Build history of the part. All positions in model axes, mm. A direction names the side the tool comes from. Round coordinates to 2 decimals unless told otherwise and drop trailing zeros. Loops run counter-clockwise (first coordinate to the right, second up) from the corner with the lowest first, then second, coordinate; pieces in that order, holes last. Notation, with made-up numbers: (-22.75, 58) - (30.25, 58) arc R14 ccw to (30.25, 64) - close; hole circle Ø4 at (77.25, 86). An arc over 180 degrees is marked (long way). Answer as CSV lines item,"result". Start each with the question number.
Autodesk Inventor part; units mm, degrees
ref_plane "YZ Plane" through (0, 0, 0) normal (1, 0, 0) x (0, 1, 0)
ref_plane "XZ Plane" through (0, 0, 0) normal (0, 1, 0) x (-1, 0, 0)
ref_plane "XY Plane" through (0, 0, 0) normal (0, 0, 1) x (1, 0, 0)
sketch "Sketch1" plane through (0, 0, 0) normal (0, 1, 0) x (-1, 0, 0)
  line L0 (56, 0) -> (-56, 0)
  line L1 (0, -49) -> (0, 49)
  line L2 (40, -20) -> (-40, -20)
  line L3 (-40, -20) -> (-40, 20)
  line L4 (-40, 20) -> (40, 20)
  line L5 (40, 20) -> (40, -20)
  line L6 (27.5, -35) -> (-27.5, -35) construction
  line L7 (-27.5, -35) -> (-27.5, 35) construction
  line L8 (-27.5, 35) -> (27.5, 35) construction
  line L9 (27.5, 35) -> (27.5, -35) construction
  point P0 (0, 0)
  dimension "d0" = 80
  dimension "d1" = 40
  dimension "d2" = 70
  dimension "d3" = 55
extrude "Extrusion1" add sketch "Sketch1" along normal blind 4
sketch "Sketch18" plane through (0, 4, 0) normal (0, 1, 0) x (1, 0, 0)
  line L0 (40, 20) -> (-40, 20)
  line L1 (-40, 20) -> (-40, -20)
  line L2 (-40, -20) -> (40, -20)
  line L3 (40, -20) -> (40, 20)
  line L4 (-40, -20) -> (40, -20)
  line L5 (40, -20) -> (40, -17)
  line L6 (40, -17) -> (-40, -17)
  line L7 (-40, -17) -> (-40, -20)
  line L8 (-40, 20) -> (-40, -20)
  line L9 (40, -20) -> (40, 20)
  line L10 (-40, -20) -> (40, -20)
  point P0 (0, 0)
  dimension "d207" = 3
extrude "Extrusion13" add sketch "Sketch18" along normal blind 10 contours L3 L2 L1 L6
sketch "Sketch19" plane through (0, 4, 0) normal (0, 1, 0) x (1, 0, 0)
  line L0 (-40, -17) -> (40, -17)
  line L1 (40, -17) -> (40, 20)
  line L2 (40, 20) -> (-40, 20)
  line L3 (-40, 20) -> (-40, -17)
  line L4 (0, 28) -> (0, -28)
  point P0 (0, 0)
  point P1 (-30, 10)
  point P2 (30, 10)
  dimension "d210" = 10
  dimension "d211" = 10
hole "Hole9" at (-30, 4, -10) at (30, 4, -10) direction (0, -1, 0) diameter 6 end through all
sketch "Sketch20" plane through (0, 4, 0) normal (0, 1, 0) x (1, 0, 0)
  circle A0 centre (-30, 10) radius 3
  line L0 (-40, -17) -> (40, -17)
  line L1 (40, -17) -> (40, 20)
  line L2 (40, 20) -> (-40, 20)
  line L3 (-40, 20) -> (-40, -17)
  line L4 (-30, -17) -> (-30, 20) construction
  line L5 (-40, 20) -> (-40, -17)
  line L6 (40, 20) -> (-40, 20)
  line L7 (40, -17) -> (-40, -17)
  line L8 (-39.3154, 10) -> (-16.7888, 10) construction
  line L9 (0, 28) -> (0, -28)
  point P0 (0, 0)
  point P1 (-37, 10)
  point P2 (-23, 10)
  point P3 (-30, 3)
  point P4 (-30, 17)
  point P5 (37, 10)
  point P6 (23, 10)
  point P7 (30, 3)
  point P8 (30, 17)
  dimension "d219" = 7
  dimension "d220" = 7
  dimension "d221" = 7
  dimension "d222" = 7
hole "Hole10" at (-37, 4, -10) at (-23, 4, -10) at (-30, 4, -3) at (-30, 4, -17) at (30, 4, -3) at (37, 4, -10) at (30, 4, -17) at (23, 4, -10) direction (0, -1, 0) diameter 2 end through all
fillet "Fillet11" radius 10 2 edges at (40, 2, -20) (-40, 2, -20)
sketch "Sketch21" plane through (40, 4, 17) normal (0, 0, -1) x (-1, 0, 0)
  line L0 (80, 0) -> (0, 0)
  line L1 (80, 0) -> (80, 10)
  line L2 (0, 10) -> (80, 10)
  line L3 (0, 0) -> (0, 10)
  point P0 (40, -4)
  point P1 (5, 5)
  point P2 (75, 5)
  dimension "d232" = 5
  dimension "d233" = 5
  dimension "d234" = 5
  dimension "d235" = 5
hole "Hole11" at (35, 9, 17) at (-35, 9, 17) direction (0, 0, 1) diameter 3 end through all
chamfer "Chamfer5" distance 4 angle 45 2 edges at (-40, 14, 18.5) (40, 14, 18.5)
fillet "Fillet12" radius 3 4 edges at (-36, 14, 18.5) (-40, 10, 18.5) (36, 14, 18.5) (40, 10, 18.5)
sketch "Sketch22" plane through (40, 4, 17) normal (0, 0, -1) x (-1, 0, 0)
  circle A0 centre (5, 5) radius 1.5
  circle A1 centre (75, 5) radius 1.5
  arc A2 (0.8787, 6.8787) -> (0, 4.7574) centre (3, 4.7574) ccw
  line L0 (0, 0) -> (0, 4.7574)
  line L1 (80, 0) -> (0, 0)
  line L2 (80, 0) -> (80, 4.7574)
  arc A3 (80, 4.7574) -> (79.1213, 6.8787) centre (77, 4.7574) ccw
  line L3 (76.8787, 9.1213) -> (79.1213, 6.8787)
  arc A4 (76.8787, 9.1213) -> (74.7574, 10) centre (74.7574, 7) ccw
  line L4 (5.2426, 10) -> (74.7574, 10)
  arc A5 (5.2426, 10) -> (3.1213, 9.1213) centre (5.2426, 7) ccw
  line L5 (0.8787, 6.8787) -> (3.1213, 9.1213)
  line L6 (10, 0) -> (70, 0)
  line L7 (20, 10) -> (60, 10)
  line L8 (60, 10) -> (60, 0)
  line L9 (60, 0) -> (20, 0)
  line L10 (20, 0) -> (20, 10)
  point P0 (40, -4)
  point P1 (40, 5)
  dimension "d247" = 5
  dimension "d248" = 40
  dimension "d256" = 40
  dimension "d257" = 10
  dimension "d258" = 20
extrude "Extrusion14" cut sketch "Sketch22" against normal up to next contours L4 L8 L1 L10
chamfer "Chamfer6" distance 4 angle 45 2 edges at (-20, 14, 18.5) (20, 14, 18.5)
fillet "Fillet13" radius 3 4 edges at (-24, 14, 18.5) (-20, 10, 18.5) (24, 14, 18.5) (20, 10, 18.5)
sketch "Sketch23" plane through (40, 4, 17) normal (0, 0, -1) x (-1, 0, 0)
  arc A0 (20, 4.7574) -> (19.1213, 6.8787) centre (17, 4.7574) ccw
  line L0 (16.8787, 9.1213) -> (19.1213, 6.8787)
  arc A1 (16.8787, 9.1213) -> (14.7574, 10) centre (14.7574, 7) ccw
  line L1 (5.2426, 10) -> (14.7574, 10)
  arc A2 (5.2426, 10) -> (3.1213, 9.1213) centre (5.2426, 7) ccw
  line L2 (0.8787, 6.8787) -> (3.1213, 9.1213)
  arc A3 (0.8787, 6.8787) -> (0, 4.7574) centre (3, 4.7574) ccw
  line L3 (0, 0) -> (0, 4.7574)
  line L4 (20, 0) -> (0, 0)
  line L5 (20, 0) -> (20, 4.7574)
  circle A4 centre (5, 5) radius 1.5
  arc A5 (60.8787, 6.8787) -> (60, 4.7574) centre (63, 4.7574) ccw
  line L6 (60, 4.7574) -> (60, 0)
  line L7 (80, 0) -> (60, 0)
  line L8 (80, 0) -> (80, 4.7574)
  arc A6 (80, 4.7574) -> (79.1213, 6.8787) centre (77, 4.7574) ccw
  line L9 (76.8787, 9.1213) -> (79.1213, 6.8787)
  arc A7 (76.8787, 9.1213) -> (74.7574, 10) centre (74.7574, 7) ccw
  line L10 (65.2426, 10) -> (74.7574, 10)
  arc A8 (65.2426, 10) -> (63.1213, 9.1213) centre (65.2426, 7) ccw
  line L11 (60.8787, 6.8787) -> (63.1213, 9.1213)
  circle A9 centre (75, 5) radius 1.5
  point P0 (40, -4)
  point P1 (15, 5)
  point P2 (65, 5)
  dimension "d265" = 5
  dimension "d266" = 5
  dimension "d267" = 5
  dimension "d268" = 5
hole "Hole13" at (25, 9, 17) at (-25, 9, 17) direction (0, 0, 1) diameter 3 end through all
chamfer "Chamfer7" distance 1 angle 45 5 edges at (0, 0, -20) (37.0711, 0, -17.0711) (40, 0, 5) (-37.0711, 0, -17.0711) (-40, 0, 5)
properties part number "body_v3"
Q1. Two-plate mould, pull along Z, no slides. Class faces 1 (the flat face through (30, 9, 17)), 2 (the cylindrical face through (29, 2, -3)), 3 (the cylindrical face through (-20.22, 9.89, 18.52)): released by +Z, released by -Z, zero draft, split by the parting line, or undercut.
Q2. Band-saw the part on A-A, the plane z = -3. List the corners of the cut face in (x, y), then the cut area to 3 significant figures.
Q3. Band-saw the part on B-B, the plane x = -28. List the corners of the cut face in (y, z), then the cut area to 3 significant figures.
Q4. Wall check: probe 1 along Z at (x, y) = (30, 2.9); probe 2 along Y at (x, z) = (25, 19.25); probe 3 along Z at (x, y) = (23, 1). Give the ranges that are in metal, low to high. Write a range as [from, to].
Q5. Tool access for faces 4 (the cylindrical face through (35.89, 13.78, 18.48)), 5 (the cylindrical face through (20.235, 9.921, 18.521)): list every direction of +Z, -Z, +X, -X, +Y, -Y with a clear straight run to the whole face (end or side of a thin tool).
Q6. Pin check, flat tips, straight feed: pin 1 Ø12 at (x, z) = (-15, 7) entering from +Y; pin 2 Ø2.5 at (x, z) = (-37, -10) entering from -Y; pin 3 Ø3 at (x, y) = (27.5, 9.5) entering from -Z. Stop position of each tip, or through.
Q7. Band-saw the part on D-D, the plane x = 9.5. List the corners of the cut face in (y, z), then the cut area to 4 significant figures.
Q8. Band-saw the part on C-C, the plane z = 12.5. List the corners of the cut face in (x, y), then the cut area to 3 significant figures.
Reported:
1,face 1,"released by -Z"
1,face 2,"undercut"
1,face 3,"zero draft"
2,outline,"(-40, 1) - (-39, 0) - (-31, 0) - (-31, 4) - (-40, 4) - close; (-29, 0) - (29, 0) - (29, 4) - (-29, 4) - close; (31, 0) - (39, 0) - (40, 1) - (40, 4) - (31, 4) - close"
2,area,"303 mm2"
3,outline,"(0, -19) - (1, -20) - (4, -20) - (4, -12.24) - (0, -12.24) - close; (0, -7.76) - (4, -7.76) - (4, 17) - (14, 17) - (14, 20) - (0, 20) - close"
3,area,"172 mm2"
4,probe 1,"z = [-20, -18], [-16, -13], [-7, -4], [-2, 20]"
4,probe 2,"y = [0, 7.5], [10.5, 13.99]"
4,probe 3,"z = [-20, -11], [-9, 20]"
5,face 4,"+Z, -Z, +X, +Y"
5,face 5,"+Z, -Z, +Y"
6,pin 1,"stops at y = 4"
6,pin 2,"stops at y = 0"
6,pin 3,"stops at z = 17"
7,outline,"(0, -19) - (1, -20) - (4, -20) - (4, 20) - (0, 20) - close"
7,area,"159.5 mm2"
8,outline,"(-40, 1) - (-39, 0) - (39, 0) - (40, 1) - (40, 4) - (-40, 4) - close"
8,area,"319 mm2"
